Model file for the job. Use its own axes, mm. Face numbers are marked on the shaded views. A direction names the side the tool comes from. Coordinates: 2 decimals unless noted, no trailing zeros. Order: outer loops, then holes, each group sorted by start corner. A loop starts at its lowest first (then second) coordinate and runs counter-clockwise, first axis right, second up.
from build123d import *

# Parameters (mm, degrees)
PAD_DEPTH          = 9
SKETCH001_W        = 26.1
SKETCH001_H        = 34.4
POCKET_DEPTH       = 3
SKETCH002_R        = 22.22
PAD001_DEPTH       = 3
SKETCH003_R        = 24.44
PAD002_DEPTH       = 3
SKETCH004_R        = 26.6
PAD003_DEPTH       = 3
SKETCH005_R        = 28
PAD004_DEPTH       = 3
SKETCH006_R        = 29
PAD005_DEPTH       = 3
SKETCH007_R        = 29
PAD006_DEPTH       = 3
SKETCH008_R        = 29
PAD007_DEPTH       = 3
SKETCH009_W        = 17
SKETCH009_H        = 24
POCKET001_DEPTH    = 3
SKETCH010_W        = 16
SKETCH010_H        = 9
POCKET002_DEPTH    = 7
SKETCH011_W        = 20
SKETCH011_H        = 10
POCKET003_DEPTH    = 3
SKETCH012_R        = 1.25
POCKET004_DEPTH    = 270.433943
POLARPATTERN_COUNT = 6
SKETCH013_W        = 3
SKETCH013_H        = 38
POCKET005_DEPTH    = 3
SKETCH014_W        = 3
SKETCH014_H        = 5
POCKET006_DEPTH    = 6


with BuildPart() as part:
    # Sketch → Pad (new body)
    with BuildSketch(Plane.XY):
        Polygon((44, 0), (22, 38.105118), (-22, 38.105118), (-44, 0), (-22, -38.105118), (22, -38.105118), align=None)
    extrude(amount=PAD_DEPTH)

    # Sketch001 (on Face8 of Pad) → Pocket (cut)
    with BuildSketch(Plane.XY.offset(9)):
        with Locations((0, -13.905118)):
            Rectangle(SKETCH001_W, SKETCH001_H)
    extrude(amount=-POCKET_DEPTH, mode=Mode.SUBTRACT)

    # Sketch002 (on Face5 of Pocket) → Pad001 (join)
    with BuildSketch(Plane.XY.offset(9)):
        Polygon((22, 38.105118), (-22, 38.105118), (-44, 0), (-22, -38.105118), (22, -38.105118), (44, 0), align=None)
        Circle(SKETCH002_R, mode=Mode.SUBTRACT)
    extrude(amount=PAD001_DEPTH)

    # Sketch003 (on Face14 of Pad001) → Pad002 (join)
    with BuildSketch(Plane.XY.offset(12)):
        Polygon((40, 0), (20, 34.641016), (-20, 34.641016), (-40, 0), (-20, -34.641016), (20, -34.641016), align=None)
        Circle(SKETCH003_R, mode=Mode.SUBTRACT)
    extrude(amount=PAD002_DEPTH)

    # Sketch004 (on Face21 of Pad002) → Pad003 (join)
    with BuildSketch(Plane.XY.offset(15)):
        Polygon((41, 0), (20.5, 35.507042), (-20.5, 35.507042), (-41, 0), (-20.5, -35.507042), (20.5, -35.507042), align=None)
        Circle(SKETCH004_R, mode=Mode.SUBTRACT)
    extrude(amount=PAD003_DEPTH)

    # Sketch005 (on Face28 of Pad003) → Pad004 (join)
    with BuildSketch(Plane.XY.offset(18)):
        Polygon((19, 32.908965), (-19, 32.908965), (-38, 0), (-19, -32.908965), (19, -32.908965), (38, 0), align=None)
        Circle(SKETCH005_R, mode=Mode.SUBTRACT)
    extrude(amount=PAD004_DEPTH)

    # Sketch006 (on Face35 of Pad004) → Pad005 (join)
    with BuildSketch(Plane.XY.offset(21)):
        Polygon((39, 0), (19.5, 33.774991), (-19.5, 33.774991), (-39, 0), (-19.5, -33.774991), (19.5, -33.774991), align=None)
        Circle(SKETCH006_R, mode=Mode.SUBTRACT)
    extrude(amount=PAD005_DEPTH)

    # Sketch007 (on Face42 of Pad005) → Pad006 (join)
    with BuildSketch(Plane.XY.offset(24)):
        Polygon((36, 0), (18, 31.176915), (-18, 31.176915), (-36, 0), (-18, -31.176915), (18, -31.176915), align=None)
        Circle(SKETCH007_R, mode=Mode.SUBTRACT)
    extrude(amount=PAD006_DEPTH)

    # Sketch008 (on Face49 of Pad006) → Pad007 (join)
    with BuildSketch(Plane.XY.offset(27)):
        Polygon((37, 0), (18.5, 32.04294), (-18.5, 32.04294), (-37, 0), (-18.5, -32.04294), (18.5, -32.04294), align=None)
        Circle(SKETCH008_R, mode=Mode.SUBTRACT)
    extrude(amount=PAD007_DEPTH)

    # Sketch009 (on Face74 of Pad007) → Pocket001 (cut)
    with BuildSketch(Plane.XY.offset(6)):
        with Locations((0, -8.705118)):
            Rectangle(SKETCH009_W, SKETCH009_H)
    extrude(amount=-POCKET001_DEPTH, mode=Mode.SUBTRACT)

    # Sketch010 (on Face12 of Pocket001) → Pocket002 (cut)
    with BuildSketch(Plane.XZ.offset(38.105118)):
        with Locations((0, 7.5)):
            Rectangle(SKETCH010_W, SKETCH010_H)
    extrude(amount=-POCKET002_DEPTH, mode=Mode.SUBTRACT)

    # Sketch011 (on Face40 of Pocket002) → Pocket003 (cut)
    with BuildSketch(Plane.XY.offset(9)):
        with Locations((0, 17.22)):
            Rectangle(SKETCH011_W, SKETCH011_H)
    extrude(amount=-POCKET003_DEPTH, mode=Mode.SUBTRACT)

    # Sketch012 (on Face93 of Pocket003) → Pocket004 (cut, through all)
    with BuildSketch(Plane.XY.offset(30)):
        with Locations((-32.33, 0)):
            Circle(SKETCH012_R)
    pocket004 = extrude(amount=-POCKET004_DEPTH, mode=Mode.SUBTRACT)

    # PolarPattern: Pocket004 ×6 about axis
    polarpattern_axis = Axis((0, 0, 30), (0, 0, 1))
    for i in range(1, POLARPATTERN_COUNT):
        add(pocket004.rotate(polarpattern_axis, i * 360 / POLARPATTERN_COUNT), mode=Mode.SUBTRACT)

    # Sketch013 (on Face45 of PolarPattern) → Pocket005 (cut)
    with BuildSketch(Plane.XY.offset(6)):
        with Locations((-11.55, -12.105118)):
            Rectangle(SKETCH013_W, SKETCH013_H)
    extrude(amount=-POCKET005_DEPTH, mode=Mode.SUBTRACT)

    # Sketch014 (on Face58 of Pocket005) → Pocket006 (cut)
    with BuildSketch(Plane.XY.offset(9)):
        with Locations((-11.55, 5.794882)):
            Rectangle(SKETCH014_W, SKETCH014_H)
    extrude(amount=-POCKET006_DEPTH, mode=Mode.SUBTRACT)


solid = part.part
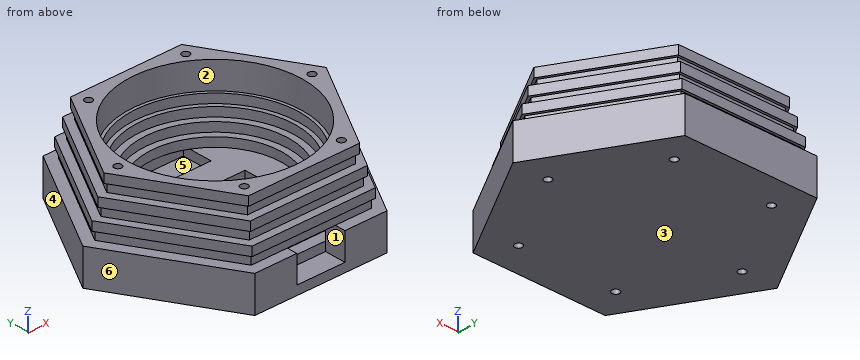
Q1. Probe line 1 (Z direction, x = 7.5, y = -31.5); line 2 (Y direction, x = 0, z = 19.4); line 3 (Z direction, x = 4, y = -32.5). List the from-to ranges inside material, lowest first.
Established:
line 1: z = 0 to 3, 12 to 24, 27 to 30
line 2: y = -32.91 to -28, 28 to 32.91
line 3: z = 0 to 3, 12 to 24
Q2. Which spindle directions (+Z, -Z, +X, -X, +Y, -Y) get a long thin tool onto all of the face, cutting with end or side? Do the marked faces 1, 2 and 3. Say none if no direction does.
Established:
face 1: -Y
face 2: +Z
face 3: -Z, +X, -X, +Y, -Y
Q3. Mould opens along Y. For the marked faces 4, 5 and 6 say: pulls with the +Y half, pulls with the -Y half, needs draft (parallel to the pull), parting line crosses it, or undercut.
Established:
face 4: pulls with the +Y half
face 5: undercut
face 6: pulls with the -Y half
Q4. Cut at B-B, the plane z = 14. List the corners of the cut face in (x, y) (3 decimals).
Established:
outline: (-40, 0) - (-20, -34.641) - (20, -34.641) - (40, 0) - (20, 34.641) - (-20, 34.641) - close; hole circle Ø2.5 at (-32.33, 0); hole circle Ø48.88 at (0, 0); hole circle Ø2.5 at (-16.165, -27.999); hole circle Ø2.5 at (-16.165, 27.999); hole circle Ø2.5 at (16.165, -27.999); hole circle Ø2.5 at (16.165, 27.999); hole circle Ø2.5 at (32.33, 0)
Q5. Drop flat-ended pins along their axis: P1, Ø4, axis at y = 15.5, z = 5, coming from the +X side; P2, Ø2, axis at y = 12, z = 18.5, coming from the -X side; P3, Ø19, axis at x = -4, y = 1, coming from the +Z side. Give the stop position or say it passes through.
Established:
P1: stops at x = 36.21
P2: stops at x = -34.57
P3: stops at z = 9
